Read the model definition and answer for the solid it produces. Units are mm, in the model's axes. A direction names the side the tool comes from. Coordinates: 2 decimals unless noted, no trailing zeros. Write each loop counter-clockwise with the first axis right and the second up, starting at its lowest first coordinate (ties: lowest second). Pieces come first, ordered by that corner, then holes.
1) Determine the mould class of faces 1 (the face through (-210, 341, -15)), 2 (the face through (-212, 341, -15)), 3 (the face through (-240, 341, -15)) for opening direction X: +X half, -X half, draft (parallel to the pull), parting line (faces both ways), or undercut.
2) Which of the six approach directions +Z, -Z, +X, -X, +Y, -Y give full straight-line access (tool end or side, diameter ignored) to faces 4 (the face through (-238, 341, -15)), 5 (the face through (-239, 290, -15))?
3) The part is cut by section B-B (z = -18.25). Determine the outline of the cut face in (x, y), then the cut area to 3 significant figures.
4) Find the intervals of material crossed by line 1 (X direction, y = 353, z = -24.75); line 2 (Z direction, x = -236.25, y = 372.5), in increasing order.
5) The part is cut by section A-A (x = -236.5). Determine the outline of the cut face in (y, z), then the cut area to 3 significant figures.
6) The part is cut by section C-C (y = 304). Determine the outline of the cut face in (x, z), then the cut area to 3 significant figures.
7) This flat-tipped pin is pushed along its axis until it touches: pin 1 Ø10 at (x, y) = (-217, 364.5) entering from +Z. Where does it stop, or does it pass through?
from build123d import *

# Parameters (mm, degrees)
SKETCH001_W   = 30
SKETCH001_H   = 30
SKETCH001_W_2 = 26
SKETCH001_H_2 = 26
PAD001_DEPTH  = 100


with BuildPart() as part:
    # Sketch001 → Pad001 (new body)
    with BuildSketch(Plane.XZ):
        with Locations((15, -15)):
            Rectangle(SKETCH001_W, SKETCH001_H)
        with Locations((15, -15)):
            Rectangle(SKETCH001_W_2, SKETCH001_H_2, mode=Mode.SUBTRACT)
    extrude(amount=PAD001_DEPTH)


with BuildPart() as part_1:
    # Body001 placement: moved
    add(part.part.moved(Location((-240, 390, 0))))


solid = part_1.part
Reported:
1. face 1: +X half
1. face 2: undercut
1. face 3: -X half
2. face 4: +Y, -Y
2. face 5: +Z, -Z, +X, -X, -Y
3. outline: (-240, 290) - (-238, 290) - (-238, 390) - (-240, 390) - close; (-212, 290) - (-210, 290) - (-210, 390) - (-212, 390) - close
3. area: 400 mm2
4. line 1: x = -240 to -238, -212 to -210
4. line 2: z = -30 to -28, -2 to 0
5. outline: (290, -30) - (390, -30) - (390, -28) - (290, -28) - close; (290, -2) - (390, -2) - (390, 0) - (290, 0) - close
5. area: 400 mm2
6. outline: (-240, -30) - (-210, -30) - (-210, 0) - (-240, 0) - close; hole (-238, -28) - (-212, -28) - (-212, -2) - (-238, -2) - close
6. area: 224 mm2
7. pin 1: stops at z = 0
